from build123d import *

# Parameters (mm, degrees)
F1_DEPTH = 110
F2_W     = 76
F2_H     = 8
F3_DEPTH = 152
F4_W     = 12
F4_H     = 57
F5_DEPTH = 152
F6_W     = 152
F6_H     = 220
F6_W_2   = 12
F6_H_2   = 57
F7_DEPTH = 145.2


# Not quite as in the source:
# - a feature names something its author has since deleted; it is built from what else it names


with BuildPart() as f1:
    # F0 (on Front) → F1 (new body, symmetric)
    with BuildSketch(Plane.XZ):
        with BuildLine():
            ThreePointArc((11.95, -69.2), (5.6567496474, -66.5932503526), (3.05, -60.3))
            Line((3.05, -60.3), (3.05, 60.3))
            ThreePointArc((3.05, 60.3), (5.6567496474, 66.5932503526), (11.95, 69.2))
            Line((11.95, 69.2), (76, 69.2))
            Line((76, 69.2), (76, 76))
            Line((76, 76), (-76, 76))
            Line((-76, 76), (-76, 69.2))
            Line((-76, 69.2), (-11.95, 69.2))
            ThreePointArc((-11.95, 69.2), (-5.6567496474, 66.5932503526), (-3.05, 60.3))
            Line((-3.05, 60.3), (-3.05, -60.3))
            ThreePointArc((-3.05, -60.3), (-5.6567496474, -66.5932503526), (-11.95, -69.2))
            Line((-11.95, -69.2), (-76, -69.2))
            Line((-76, -69.2), (-76, -76))
            Line((-76, -76), (76, -76))
            Line((76, -76), (76, -69.2))
            Line((76, -69.2), (11.95, -69.2))
        make_face()
    extrude(amount=F1_DEPTH, both=True)

    # F2 (on face) → F3 (join)
    with BuildSketch(Plane.XY.offset(76)):
        with Locations((-38, 0)):
            Rectangle(F2_W, F2_H)
    extrude(amount=-F3_DEPTH)

    # F4 (on face) → F5 (cut)
    with BuildSketch(Plane.XY.offset(76)):
        with BuildLine():
            ThreePointArc((-48.16667, 90.7352813742), (-45.2167956289, 86.9404157598), (-44.16667, 82.25))
            Line((-44.16667, 82.25), (-44.16667, 25.25))
            ThreePointArc((-44.16667, 25.25), (-45.2167956289, 20.5595842402), (-48.16667, 16.7647186258))
            Line((-48.16667, 16.7647186258), (-48.16667, 2.5))
            Line((-48.16667, 2.5), (-30.16667, 2.5))
            Line((-30.16667, 2.5), (-30.16667, 16.7647186258))
            ThreePointArc((-30.16667, 16.7647186258), (-33.1165443711, 20.5595842402), (-34.16667, 25.25))
            Line((-34.16667, 25.25), (-34.16667, 82.25))
            ThreePointArc((-34.16667, 82.25), (-33.1165443711, 86.9404157598), (-30.16667, 90.7352813742))
            Line((-30.16667, 90.7352813742), (-30.16667, 105))
            Line((-30.16667, 105), (-48.16667, 105))
            Line((-48.16667, 105), (-48.16667, 90.7352813742))
        make_face()
        with BuildLine():
            Line((-71.16667, 2.5), (-53.16667, 2.5))
            Line((-53.16667, 2.5), (-53.16667, 16.7647186258))
            ThreePointArc((-53.16667, 16.7647186258), (-56.1165443711, 20.5595842402), (-57.16667, 25.25))
            Line((-57.16667, 25.25), (-57.16667, 82.25))
            ThreePointArc((-57.16667, 82.25), (-56.1165443711, 86.9404157598), (-53.16667, 90.7352813742))
            Line((-53.16667, 90.7352813742), (-53.16667, 105))
            Line((-53.16667, 105), (-71.16667, 105))
            Line((-71.16667, 105), (-71.16667, 90.7352813742))
            ThreePointArc((-71.16667, 90.7352813742), (-68.2167956289, 86.9404157598), (-67.16667, 82.25))
            Line((-67.16667, 82.25), (-67.16667, 25.25))
            ThreePointArc((-67.16667, 25.25), (-68.2167956289, 20.5595842402), (-71.16667, 16.7647186258))
            Line((-71.16667, 16.7647186258), (-71.16667, 2.5))
        make_face()
        with Locations((31, 55)):
            Rectangle(F4_W, F4_H)
        with Locations((48, 55)):
            Rectangle(F4_W, F4_H)
        with Locations((65, 55)):
            Rectangle(F4_W, F4_H)
        with Locations((31, -55)):
            Rectangle(F4_W, F4_H)
        with Locations((48, -55)):
            Rectangle(F4_W, F4_H)
        with Locations((65, -55)):
            Rectangle(F4_W, F4_H)
        with BuildLine():
            Line((-71.16667, -105), (-53.16667, -105))
            Line((-53.16667, -105), (-53.16667, -90.7352813742))
            ThreePointArc((-53.16667, -90.7352813742), (-56.1165443711, -86.9404157598), (-57.16667, -82.25))
            Line((-57.16667, -82.25), (-57.16667, -25.25))
            ThreePointArc((-57.16667, -25.25), (-56.1165443711, -20.5595842402), (-53.16667, -16.7647186258))
            Line((-53.16667, -16.7647186258), (-53.16667, -2.5))
            Line((-53.16667, -2.5), (-71.16667, -2.5))
            Line((-71.16667, -2.5), (-71.16667, -16.7647186258))
            ThreePointArc((-71.16667, -16.7647186258), (-68.2167956289, -20.5595842402), (-67.16667, -25.25))
            Line((-67.16667, -25.25), (-67.16667, -82.25))
            ThreePointArc((-67.16667, -82.25), (-68.2167956289, -86.9404157598), (-71.16667, -90.7352813742))
            Line((-71.16667, -90.7352813742), (-71.16667, -105))
        make_face()
        with BuildLine():
            ThreePointArc((-48.16667, -16.7647186258), (-45.2167956289, -20.5595842402), (-44.16667, -25.25))
            Line((-44.16667, -25.25), (-44.16667, -82.25))
            ThreePointArc((-44.16667, -82.25), (-45.2167956289, -86.9404157598), (-48.16667, -90.7352813742))
            Line((-48.16667, -90.7352813742), (-48.16667, -105))
            Line((-48.16667, -105), (-30.16667, -105))
            Line((-30.16667, -105), (-30.16667, -90.7352813742))
            ThreePointArc((-30.16667, -90.7352813742), (-33.1165443711, -86.9404157598), (-34.16667, -82.25))
            Line((-34.16667, -82.25), (-34.16667, -25.25))
            ThreePointArc((-34.16667, -25.25), (-33.1165443711, -20.5595842402), (-30.16667, -16.7647186258))
            Line((-30.16667, -16.7647186258), (-30.16667, -2.5))
            Line((-30.16667, -2.5), (-48.16667, -2.5))
            Line((-48.16667, -2.5), (-48.16667, -16.7647186258))
        make_face()
    extrude(amount=-F5_DEPTH, mode=Mode.SUBTRACT)

    # F6 (on face) → F7 (cut)
    with BuildSketch(Plane(origin=(0, 0, -76), x_dir=(1, 0, 0), z_dir=(0, 0, -1))):
        Rectangle(F6_W, F6_H)
        with BuildLine():
            Line((-67.16667, -82.25), (-67.16667, -25.25))
            ThreePointArc((-67.16667, -25.25), (-68.2167956289, -20.5595842402), (-71.16667, -16.7647186258))
            Line((-71.16667, -16.7647186258), (-71.16667, -2.5))
            Line((-71.16667, -2.5), (-53.16667, -2.5))
            Line((-53.16667, -2.5), (-53.16667, -16.7647186258))
            ThreePointArc((-53.16667, -16.7647186258), (-56.1165443711, -20.5595842402), (-57.16667, -25.25))
            Line((-57.16667, -25.25), (-57.16667, -82.25))
            ThreePointArc((-57.16667, -82.25), (-56.1165443711, -86.9404157598), (-53.16667, -90.7352813742))
            Line((-53.16667, -90.7352813742), (-53.16667, -105))
            Line((-53.16667, -105), (-71.16667, -105))
            Line((-71.16667, -105), (-71.16667, -90.7352813742))
            ThreePointArc((-71.16667, -90.7352813742), (-68.2167956289, -86.9404157598), (-67.16667, -82.25))
        make_face(mode=Mode.SUBTRACT)
        with BuildLine():
            Line((-30.16667, -105), (-48.16667, -105))
            Line((-48.16667, -105), (-48.16667, -90.7352813742))
            ThreePointArc((-48.16667, -90.7352813742), (-45.2167956289, -86.9404157598), (-44.16667, -82.25))
            Line((-44.16667, -82.25), (-44.16667, -25.25))
            ThreePointArc((-44.16667, -25.25), (-45.2167956289, -20.5595842402), (-48.16667, -16.7647186258))
            Line((-48.16667, -16.7647186258), (-48.16667, -2.5))
            Line((-48.16667, -2.5), (-30.16667, -2.5))
            Line((-30.16667, -2.5), (-30.16667, -16.7647186258))
            ThreePointArc((-30.16667, -16.7647186258), (-33.1165443711, -20.5595842402), (-34.16667, -25.25))
            Line((-34.16667, -25.25), (-34.16667, -82.25))
            ThreePointArc((-34.16667, -82.25), (-33.1165443711, -86.9404157598), (-30.16667, -90.7352813742))
            Line((-30.16667, -90.7352813742), (-30.16667, -105))
        make_face(mode=Mode.SUBTRACT)
        with Locations((31, -55)):
            Rectangle(F6_W_2, F6_H_2, mode=Mode.SUBTRACT)
        with Locations((48, -55)):
            Rectangle(F6_W_2, F6_H_2, mode=Mode.SUBTRACT)
        with Locations((65, -55)):
            Rectangle(F6_W_2, F6_H_2, mode=Mode.SUBTRACT)
        with BuildLine():
            ThreePointArc((-67.16667, 82.25), (-68.2167956289, 86.9404157598), (-71.16667, 90.7352813742))
            Line((-71.16667, 90.7352813742), (-71.16667, 105))
            Line((-71.16667, 105), (-53.16667, 105))
            Line((-53.16667, 105), (-53.16667, 90.7352813742))
            ThreePointArc((-53.16667, 90.7352813742), (-56.1165443711, 86.9404157598), (-57.16667, 82.25))
            Line((-57.16667, 82.25), (-57.16667, 25.25))
            ThreePointArc((-57.16667, 25.25), (-56.1165443711, 20.5595842402), (-53.16667, 16.7647186258))
            Line((-53.16667, 16.7647186258), (-53.16667, 2.5))
            Line((-53.16667, 2.5), (-71.16667, 2.5))
            Line((-71.16667, 2.5), (-71.16667, 16.7647186258))
            ThreePointArc((-71.16667, 16.7647186258), (-68.2167956289, 20.5595842402), (-67.16667, 25.25))
            Line((-67.16667, 25.25), (-67.16667, 82.25))
        make_face(mode=Mode.SUBTRACT)
        with BuildLine():
            Line((-30.16667, 2.5), (-48.16667, 2.5))
            Line((-48.16667, 2.5), (-48.16667, 16.7647186258))
            ThreePointArc((-48.16667, 16.7647186258), (-45.2167956289, 20.5595842402), (-44.16667, 25.25))
            Line((-44.16667, 25.25), (-44.16667, 82.25))
            ThreePointArc((-44.16667, 82.25), (-45.2167956289, 86.9404157598), (-48.16667, 90.7352813742))
            Line((-48.16667, 90.7352813742), (-48.16667, 105))
            Line((-48.16667, 105), (-30.16667, 105))
            Line((-30.16667, 105), (-30.16667, 90.7352813742))
            ThreePointArc((-30.16667, 90.7352813742), (-33.1165443711, 86.9404157598), (-34.16667, 82.25))
            Line((-34.16667, 82.25), (-34.16667, 25.25))
            ThreePointArc((-34.16667, 25.25), (-33.1165443711, 20.5595842402), (-30.16667, 16.7647186258))
            Line((-30.16667, 16.7647186258), (-30.16667, 2.5))
        make_face(mode=Mode.SUBTRACT)
        with Locations((31, 55)):
            Rectangle(F6_W_2, F6_H_2, mode=Mode.SUBTRACT)
        with Locations((48, 55)):
            Rectangle(F6_W_2, F6_H_2, mode=Mode.SUBTRACT)
        with Locations((65, 55)):
            Rectangle(F6_W_2, F6_H_2, mode=Mode.SUBTRACT)
    extrude(amount=-F7_DEPTH, mode=Mode.SUBTRACT)


solid = f1.part
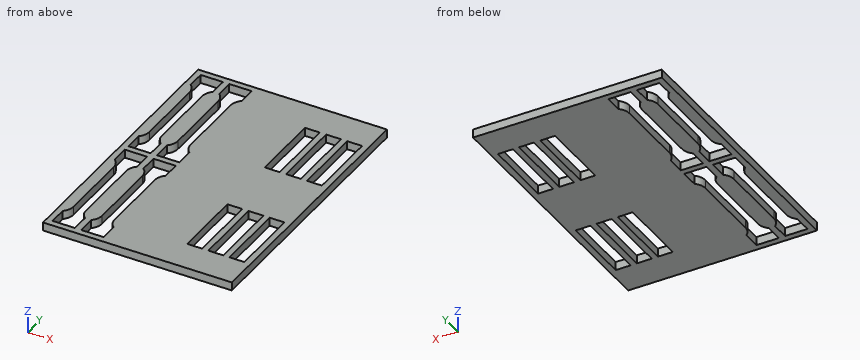
Read the model definition and answer for the solid it produces. Units are mm, in the model's axes. Coordinates: 2 decimals unless noted, no trailing zeros. Loops run counter-clockwise (first coordinate to the right, second up) from the corner with the lowest first, then second, coordinate; pieces in that order, holes last.
Q1. The part is cut by section C-C on x = 62.5. Write down the section's boundary in (y, z), and give its area (3 significant figures).
Q2. The part is cut by section D-D on z = 70.25. Give the number of separate pieces and of enclosed holes in the cut face, and give its area (3 significant figures).
Q3. The part is cut by section A-A on y = -97. Write down the section's boundary in (x, z), and give its area (3 significant figures).
Q4. Consider probe 1 along Y at (x, z) = (65.5, 72.75); probe 2 along X at (y, z) = (50, 70.75); probe 3 along X at (y, z) = (-96, 75). Determine where each line is inside the solid, lowest interval first.
Q5. The part is cut by section B-B on y = 36.5. Write down the section's boundary in (x, z).
Results below:
1. outline: (-110, 69.2) - (-83.5, 69.2) - (-83.5, 76) - (-110, 76) - close; (-26.5, 69.2) - (26.5, 69.2) - (26.5, 76) - (-26.5, 76) - close; (83.5, 69.2) - (110, 69.2) - (110, 76) - (83.5, 76) - close
1. area: 721 mm2
2. separate pieces: 1
2. enclosed holes: 10
2. area: 24,200 mm2
3. outline: (-76, 69.2) - (-71.17, 69.2) - (-71.17, 76) - (-76, 76) - close; (-53.17, 69.2) - (-48.17, 69.2) - (-48.17, 76) - (-53.17, 76) - close; (-30.17, 69.2) - (76, 69.2) - (76, 76) - (-30.17, 76) - close
3. area: 789 mm2
4. probe 1: y = -110 to -83.5, -26.5 to 26.5, 83.5 to 110
4. probe 2: x = -76 to -67.17, -57.17 to -44.17, -34.17 to 25, 37 to 42, 54 to 59, 71 to 76
4. probe 3: x = -76 to -71.17, -53.17 to -48.17, -30.17 to 76
5. outline: (-76, 69.2) - (-67.17, 69.2) - (-67.17, 76) - (-76, 76) - close; (-57.17, 69.2) - (-44.17, 69.2) - (-44.17, 76) - (-57.17, 76) - close; (-34.17, 69.2) - (25, 69.2) - (25, 76) - (-34.17, 76) - close; (37, 69.2) - (42, 69.2) - (42, 76) - (37, 76) - close; (54, 69.2) - (59, 69.2) - (59, 76) - (54, 76) - close; (71, 69.2) - (76, 69.2) - (76, 76) - (71, 76) - close
